Build history of the part. All positions in model axes, mm. A direction names the side the tool comes from. Give positions to 0.01 mm unless a question says otherwise; leave off trailing zeros. Order: outer loops, then holes, each group sorted by start corner. A loop starts at its lowest first (then second) coordinate and runs counter-clockwise, first axis right, second up. Notation, with made-up numbers: (49, 18) -> (99, 18) arc R35 ccw to (99, 53) -> close; hole circle Ø5 at (26.5, -37). An arc over 180 degrees is marked (long way). Use a Markdown table: item, result. Add a question column.
```python
from build123d import *

# Parameters (mm, degrees)
F1_DEPTH = 2.5
F2_DEPTH = 23
F3_R     = 3
F4_R     = 1
F5_R     = 3


with BuildPart() as f1:
    # F0 (on Top) → F1 (new body)
    with BuildSketch(Plane.XY):
        with BuildLine():
            Line((80.771052, 39.371213), (-79.228948, 39.371213))
            ThreePointArc((-79.228948, 39.371213), (-84.532249, 37.174514), (-86.728948, 31.871213))
            Line((-86.728948, 31.871213), (-86.728948, -20.128787))
            ThreePointArc((-86.728948, -20.128787), (-84.532249, -25.432087), (-79.228948, -27.628787))
            Line((-79.228948, -27.628787), (80.771052, -27.628787))
            ThreePointArc((80.771052, -27.628787), (86.074353, -25.432087), (88.271052, -20.128787))
            Line((88.271052, -20.128787), (88.271052, 31.871213))
            ThreePointArc((88.271052, 31.871213), (86.074353, 37.174514), (80.771052, 39.371213))
        make_face()
        with BuildLine():
            ThreePointArc((-84.228948, 31.871213), (-82.764482, 35.406747), (-79.228948, 36.871213))
            Line((-79.228948, 36.871213), (80.771052, 36.871213))
            ThreePointArc((80.771052, 36.871213), (84.306586, 35.406747), (85.771052, 31.871213))
            Line((85.771052, 31.871213), (85.771052, -20.128787))
            ThreePointArc((85.771052, -20.128787), (84.306586, -23.66432), (80.771052, -25.128787))
            Line((80.771052, -25.128787), (-79.228948, -25.128787))
            ThreePointArc((-79.228948, -25.128787), (-82.764482, -23.66432), (-84.228948, -20.128787))
            Line((-84.228948, -20.128787), (-84.228948, 31.871213))
        make_face(mode=Mode.SUBTRACT)
        with BuildLine():
            Line((80.771052, 36.871213), (-79.228948, 36.871213))
            ThreePointArc((-79.228948, 36.871213), (-82.764482, 35.406747), (-84.228948, 31.871213))
            Line((-84.228948, 31.871213), (-84.228948, -20.128787))
            ThreePointArc((-84.228948, -20.128787), (-82.764482, -23.66432), (-79.228948, -25.128787))
            Line((-79.228948, -25.128787), (80.771052, -25.128787))
            ThreePointArc((80.771052, -25.128787), (84.306586, -23.66432), (85.771052, -20.128787))
            Line((85.771052, -20.128787), (85.771052, 31.871213))
            ThreePointArc((85.771052, 31.871213), (84.306586, 35.406747), (80.771052, 36.871213))
        make_face()
    extrude(amount=F1_DEPTH)

    # F0 (on Top) → F2 (join)
    with BuildSketch(Plane.XY):
        with BuildLine():
            Line((80.771052, 39.371213), (-79.228948, 39.371213))
            ThreePointArc((-79.228948, 39.371213), (-84.532249, 37.174514), (-86.728948, 31.871213))
            Line((-86.728948, 31.871213), (-86.728948, -20.128787))
            ThreePointArc((-86.728948, -20.128787), (-84.532249, -25.432087), (-79.228948, -27.628787))
            Line((-79.228948, -27.628787), (80.771052, -27.628787))
            ThreePointArc((80.771052, -27.628787), (86.074353, -25.432087), (88.271052, -20.128787))
            Line((88.271052, -20.128787), (88.271052, 31.871213))
            ThreePointArc((88.271052, 31.871213), (86.074353, 37.174514), (80.771052, 39.371213))
        make_face()
        with BuildLine():
            ThreePointArc((-84.228948, 31.871213), (-82.764482, 35.406747), (-79.228948, 36.871213))
            Line((-79.228948, 36.871213), (80.771052, 36.871213))
            ThreePointArc((80.771052, 36.871213), (84.306586, 35.406747), (85.771052, 31.871213))
            Line((85.771052, 31.871213), (85.771052, -20.128787))
            ThreePointArc((85.771052, -20.128787), (84.306586, -23.66432), (80.771052, -25.128787))
            Line((80.771052, -25.128787), (-79.228948, -25.128787))
            ThreePointArc((-79.228948, -25.128787), (-82.764482, -23.66432), (-84.228948, -20.128787))
            Line((-84.228948, -20.128787), (-84.228948, 31.871213))
        make_face(mode=Mode.SUBTRACT)
    extrude(amount=F2_DEPTH)

    # F3
    f3_edges = [f1.edges().sort_by_distance(p)[0] for p in [
        (0.771052, 39.371213, 0),
        (-84.532249, 37.174514, 0),
        (-86.728948, 5.871213, 0),
        (-84.532249, -25.432087, 0),
        (0.771052, -27.628787, 0),
        (86.074353, -25.432087, 0),
        (88.271052, 5.871213, 0),
        (86.074353, 37.174514, 0),
    ]]
    fillet(f3_edges, radius=F3_R)

    # F4
    f4_edges = [f1.edges().sort_by_distance(p)[0] for p in [
        (0.771052, 39.371213, 23),
        (-84.532249, 37.174514, 23),
        (-86.728948, 5.871213, 23),
        (-84.532249, -25.432087, 23),
        (0.771052, -27.628787, 23),
        (86.074353, -25.432087, 23),
        (88.271052, 5.871213, 23),
        (86.074353, 37.174514, 23),
        (-84.228948, 5.871213, 23),
        (-82.764482, 35.406747, 23),
        (0.771052, 36.871213, 23),
        (84.306586, 35.406747, 23),
        (85.771052, 5.871213, 23),
        (84.306586, -23.66432, 23),
        (0.771052, -25.128787, 23),
        (-82.764482, -23.66432, 23),
    ]]
    fillet(f4_edges, radius=F4_R)

    # F5
    f5_edges = [f1.edges().sort_by_distance(p)[0] for p in [
        (0.771052, -25.128787, 2.5),
        (84.306586, -23.66432, 2.5),
        (0.771052, 36.871213, 2.5),
        (84.306586, 35.406747, 2.5),
        (-82.764482, -23.66432, 2.5),
        (-84.228948, 5.871213, 2.5),
        (-82.764482, 35.406747, 2.5),
        (85.771052, 5.871213, 2.5),
    ]]
    fillet(f5_edges, radius=F5_R)


solid = f1.part
```
(1) Pin check, flat tip, straight feed: pin 1 Ø6 at (x, y) = (-59.5, 20.5) entering from +Z. Stop position of the tip, or through.
(2) Band-saw the part on B-B on x = 43.5. Give the cut face in (y, z).
(3) Band-saw the part on C-C on y = -16. Give the cut face in (x, z), plus the area to 3 significant figures.
(4) Mould opens along Y. For faces 3 (the face through (-86.729, 6, 12)), 4 (the face through (-84.229, 6, 14)), 5 (the face through (-84.59, -25.373, 12.367)), 6 (the face through (-0.349, 38.516, 0.902)) say: released by +Y, released by -Y, zero draft, split by the parting line, or undercut.
(5) Wall check: probe 1 along Y at (x, z) = (52, 7); probe 2 along X at (y, z) = (-19, 20.75); probe 3 along Z at (x, y) = (-27.5, -6). Give the ranges that are in metal, low to high.
(6) Band-saw the part on A-A on z = 9.5. Give the cut face in (x, y), plus the area to 3 significant figures.
(7) Tool access for faces 1 (the face through (85.771, 6, 14)), 2 (the face through (0, 6, 0)): list every direction of +Z, -Z, +X, -X, +Y, -Y with a clear straight run to the whole face (end or side of a thin tool).
Response:
| question | item | result |
|---|---|---|
| 1 | pin 1 | stops at z = 2.5 |
| 2 | outline | (-27.63, 3) arc R3 ccw to (-24.63, 0) -> (36.37, 0) arc R3 ccw to (39.37, 3) -> (39.37, 22) arc R1 ccw to (38.37, 23) -> (37.87, 23) arc R1 ccw to (36.87, 22) -> (36.87, 5.5) arc R3 cw to (33.87, 2.5) -> (-22.13, 2.5) arc R3 cw to (-25.13, 5.5) -> (-25.13, 22) arc R1 ccw to (-26.13, 23) -> (-26.63, 23) arc R1 ccw to (-27.63, 22) -> close |
| 3 | outline | (-86.73, 3) arc R3 ccw to (-83.73, 0) -> (85.27, 0) arc R3 ccw to (88.27, 3) -> (88.27, 22) arc R1 ccw to (87.27, 23) -> (86.77, 23) arc R1 ccw to (85.77, 22) -> (85.77, 5.5) arc R3 cw to (82.77, 2.5) -> (-81.23, 2.5) arc R3 cw to (-84.23, 5.5) -> (-84.23, 22) arc R1 ccw to (-85.23, 23) -> (-85.73, 23) arc R1 ccw to (-86.73, 22) -> close |
| 3 | area | 539 mm² |
| 4 | face 3 | zero draft |
| 4 | face 4 | undercut |
| 4 | face 5 | released by -Y |
| 4 | face 6 | released by +Y |
| 5 | probe 1 | y = -27.63 to -25.13, 36.87 to 39.37 |
| 5 | probe 2 | x = -86.73 to -84.23, 85.77 to 88.27 |
| 5 | probe 3 | z = 0 to 2.5 |
| 6 | outline | (-86.73, -20.13) arc R7.5 ccw to (-79.23, -27.63) -> (80.77, -27.63) arc R7.5 ccw to (88.27, -20.13) -> (88.27, 31.87) arc R7.5 ccw to (80.77, 39.37) -> (-79.23, 39.37) arc R7.5 ccw to (-86.73, 31.87) -> close; hole (-84.23, -20.13) arc R5 ccw to (-79.23, -25.13) -> (80.77, -25.13) arc R5 ccw to (85.77, -20.13) -> (85.77, 31.87) arc R5 ccw to (80.77, 36.87) -> (-79.23, 36.87) arc R5 ccw to (-84.23, 31.87) -> close |
| 6 | area | 1,160 mm² |
| 7 | face 1 | +Z |
| 7 | face 2 | -Z, +X, -X, +Y, -Y |
